Geometry check sheet. Reference: the model listing, model coordinates, mm. A direction names the side the tool comes from. Coordinates: 2 decimals unless noted, no trailing zeros. Write each loop counter-clockwise with the first axis right and the second up, starting at its lowest first coordinate (ties: lowest second). Pieces come first, ordered by that corner, then holes. Notation, with made-up numbers: M 17.5,75 L 73.5,75 A19 ccw 73.5,84 Z; hole C -26,46.5 d9. An arc over 180 degrees is marked long. Put each result on its own line as item: value. Start each with the question number.
1) Cross-section at A-A on x = 0. Record the cut outline in (y, z), plus the area to 3 significant figures.
2) Set-up check for faces 1 (the flat face through (-1, 65, 0)), 2 (the cylindrical face through (66.64, 19.44, 15.06)): record each of +Z, -Z, +X, -X, +Y, -Y from which the full face is reachable in a straight line by a thin tool's end or side.
3) Scan lines: line 1 along Z through (x, y) = (-73, 40); line 2 along X through (y, z) = (6.5, 26.75); line 3 along X through (y, z) = (16.5, 20.25). Record each from-to range of solid material in increasing order.
4) Gauge pin test, flat ends, axial feed: pin 1 (12 mm diameter, centred on x = 64.5, z = 23, fed in from -Y); pin 2 (5 mm diameter, centred on y = 68, z = 10.5, fed in from +X); pin 3 (1.5 mm diameter, centred on y = 20, z = 9, fed in from +X). Record the tip position at first contact, or that the pin passes through.
5) Mould release check, pull along X, two halves, no side actions. Record for faces 3 (the flat face through (-74, 12, 27.94)), 4 (the cylindrical face through (-81.786, 19.437, 15.062)), 5 (the cylindrical face through (1.95, 88.88, 1.25)): released by +X, released by -X, zero draft, split by the parting line, or undercut.
6) Cross-section at B-B on y = 8.5. Record the cut outline in (x, z), plus the area to 3 significant figures.
7) Cross-section at C-C on z = 5.5. Record the cut outline in (x, y).
8) Cross-section at D-D on y = 73.5. Record the cut outline in (x, z).
from build123d import *

# Parameters (mm, degrees)
F1_DEPTH = 2.54
F2_R     = 10.541
F3_DEPTH = 25.4


with BuildPart() as f1:
    # F0 (on Top) → F1 (new body)
    with BuildSketch(Plane.XY):
        with BuildLine():
            Line((63.5, 0), (88.9, 0))
            ThreePointArc((88.9, 0), (0, 88.9), (-88.9, 0))
            Line((-88.9, 0), (-63.5, 0))
            ThreePointArc((-63.5, 0), (0, 63.5), (63.5, 0))
        make_face()
    extrude(amount=F1_DEPTH)

    # F2 (on face) → F3 (join)
    with BuildSketch(Plane.XY.offset(2.54)):
        with Locations((0, 75.959727)):
            Circle(F2_R)
        with Locations((-74.016793, 12.313276)):
            Circle(F2_R)
        with Locations((74.406557, 12.313276)):
            Circle(F2_R)
    extrude(amount=F3_DEPTH)


solid = f1.part
Answer key:
1. outline: M 63.5,0 L 88.9,0 L 88.9,2.54 L 86.5,2.54 L 86.5,27.94 L 65.42,27.94 L 65.42,2.54 L 63.5,2.54 Z
1. area: 600 mm²
2. face 1: -Z, +X, -X, +Y, -Y
2. face 2: +Z
3. line 1: z = 0 to 2.54
3. line 2: x = -82.81 to -65.22, 65.61 to 83.2
3. line 3: x = -83.69 to -64.34, 64.73 to 84.08
4. pin 1: stops at y = 2.52
4. pin 2: stops at x = 9.02
4. pin 3: stops at x = 82.34
5. face 3: zero draft
5. face 4: undercut
5. face 5: split by the parting line
6. outline: M -88.49,0 L -62.93,0 L -62.93,2.54 L -64.19,2.54 L -64.19,27.94 L -83.84,27.94 L -83.84,2.54 L -88.49,2.54 Z; M 62.93,0 L 88.49,0 L 88.49,2.54 L 84.23,2.54 L 84.23,27.94 L 64.58,27.94 L 64.58,2.54 L 62.93,2.54 Z
6. area: 1,130 mm²
7. outline: C -74.02,12.31 d21.08; C 0,75.96 d21.08; C 74.41,12.31 d21.08
8. outline: M -50.01,0 L 50.01,0 L 50.01,2.54 L 10.25,2.54 L 10.25,27.94 L -10.25,27.94 L -10.25,2.54 L -50.01,2.54 Z
